Drawing for the job (mm, zero at the part's lowest x, y, z). A direction names the side the tool comes from. Coordinates: 2 decimals unless noted, no trailing zeros. Loops run counter-clockwise (first coordinate to the right, second up) from the corner with the lowest first, then second, coordinate; pieces in that order, holes last. Notation, with made-up numbers: (73.25, 38.25) - (95.25, 38.25) arc R12 ccw to (95.25, 55.25) - close; hole circle Ø1 at (68.5, 7.25). An arc over 180 degrees is marked (long way). Put each result on its own line as item: value.
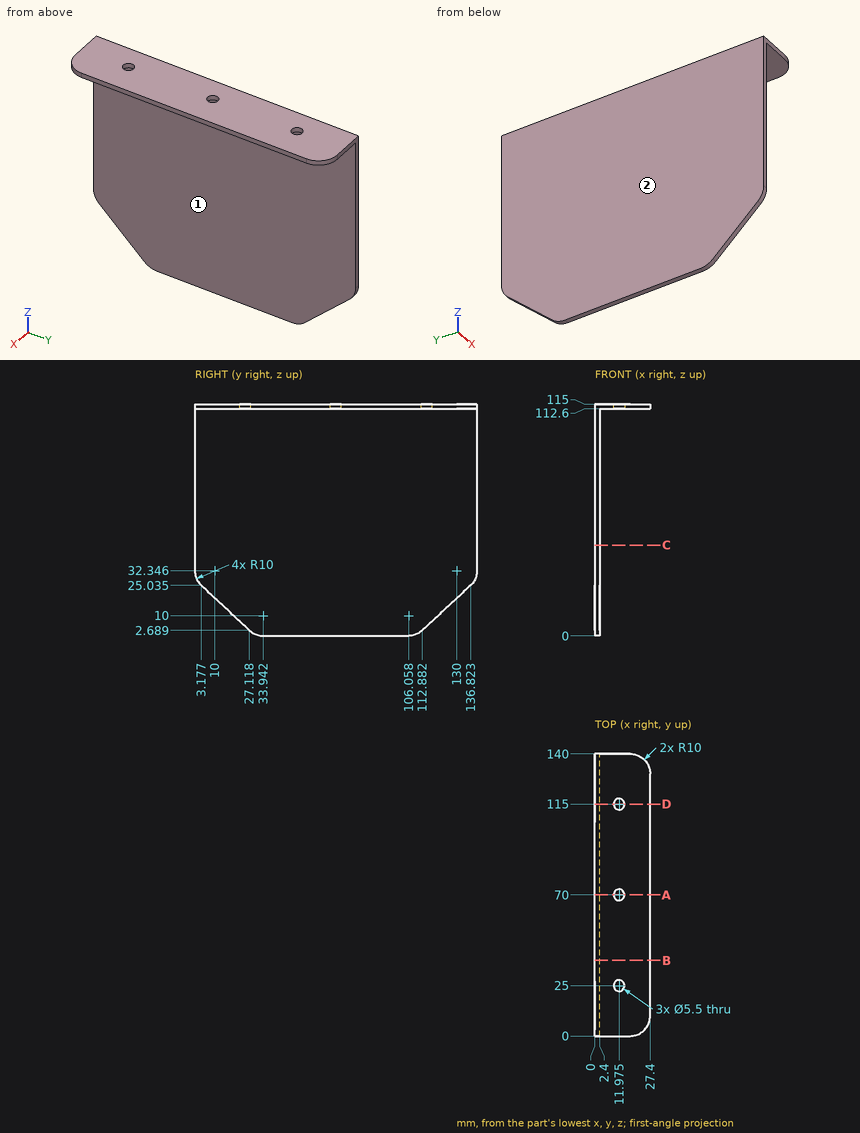
Q1. Slice it at A-A, the plane y = 70. Give the cut face in (x, z) (1 decimal).
Determined:
outline: (0, 0) - (2.4, 0) - (2.4, 112.6) - (9.2, 112.6) - (9.2, 115) - (0, 115) - close; (14.7, 112.6) - (27.4, 112.6) - (27.4, 115) - (14.7, 115) - close
Q2. Slice it at D-D, the plane y = 115. Give the cut face in (x, z) (1 decimal).
Determined:
outline: (0, 4.7) - (2.4, 4.7) - (2.4, 112.6) - (9.2, 112.6) - (9.2, 115) - (0, 115) - close; (14.7, 112.6) - (27.4, 112.6) - (27.4, 115) - (14.7, 115) - close
Q3. Slice it at C-C, the plane z = 45. Give the cut face in (x, y).
Determined:
outline: (0, 0) - (2.4, 0) - (2.4, 140) - (0, 140) - close
Q4. Slice it at B-B, the plane y = 37.5. Give the cut face in (x, z).
Determined:
outline: (0, 0) - (2.4, 0) - (2.4, 112.6) - (27.4, 112.6) - (27.4, 115) - (0, 115) - close
Q5. Tool access for the marked faces 1 and 2: list every direction of +Z, -Z, +X, -X, +Y, -Y with a clear straight run to the whole face (end or side of a thin tool).
Determined:
face 1: -Z, +X, +Y, -Y
face 2: +Z, -Z, -X, +Y, -Y
Q6. Wall check: L1, parallel to X at y = 70, z = 113 (1 decimal); L2, parallel to Z at x = 12.75, y = 29; L3, parallel to X at y = 120.5, z = 78. Give the ranges that are in metal, low to high. Write a range as from..to.
Determined:
L1: 0..9.2, 14.7..27.4
L2: 112.6..115
L3: 0..2.4
Q7. Pin check, flat tips, straight feed: pin 1 Ø4 at (x, y) = (20.5, 109.5) entering from -Z; pin 2 Ø3.5 at (x, y) = (11.97, 25) entering from -Z. Stop position of each tip, or through.
Determined:
pin 1: z = 112.6
pin 2: through
